```python
from build123d import *

# Parameters (mm, degrees)
SKETCH1_R                    = 16.891
SKETCH1_R_2                  = 7.9375
BOSS_EXTRUDE1_DEPTH          = 12.7
SKETCH2_R                    = 20.6375
CUT_EXTRUDE1_DEPTH           = 7.3914
CHAMFER1_SIZE                = 0.254
SKETCH4_R                    = 2.1844
CUT_EXTRUDE2_DEPTH           = 6.3086
CHAMFER2_SIZE                = 0.254
CIRPATTERN1_COUNT            = 6
CHAMFER2_OF_CIRPATTERN1_SIZE = 0.254


with BuildPart() as part:
    # Sketch1 → Boss-Extrude1 (new body)
    with BuildSketch(Plane(origin=(0, 0, 0), x_dir=(1, 0, 0), z_dir=(0, 1, 0))):
        Circle(SKETCH1_R)
        Circle(SKETCH1_R_2, mode=Mode.SUBTRACT)
    extrude(amount=BOSS_EXTRUDE1_DEPTH)

    # Sketch2 → Cut-Extrude1 (cut)
    with BuildSketch(Plane(origin=(0, 12.7, 0), x_dir=(1, 0, 0), z_dir=(0, 1, 0))):
        Circle(SKETCH2_R)
    extrude(amount=-CUT_EXTRUDE1_DEPTH, mode=Mode.SUBTRACT)

    # Chamfer1
    chamfer1_edges = [part.edges().sort_by_distance(p)[0] for p in [
        (-16.891, 5.3086, 0),
        (-16.891, 0, 0),
    ]]
    chamfer(chamfer1_edges, length=CHAMFER1_SIZE)

    # Sketch3 → Cut-Revolve1 (revolve, cut)
    with BuildSketch(Plane.XY):
        Polygon((-10.7188, 0), (-10.7188, 1.2446), (-9.144, 0.6604), (-9.144, 1.27), (0, 1.27), (0, 0), align=None)
    revolve(axis=Axis((0, 12.7, 0), (0, -1, 0)), mode=Mode.SUBTRACT)

    # Sketch4 → Cut-Extrude2 (cut, through all)
    with BuildSketch(Plane(origin=(0, 5.3086, 0), x_dir=(1, 0, 0), z_dir=(0, 1, 0))):
        with Locations((0, 13.4874)):
            Circle(SKETCH4_R)
    cut_extrude2 = extrude(amount=-CUT_EXTRUDE2_DEPTH, mode=Mode.SUBTRACT)

    # Chamfer2
    chamfer2_edges = [part.edges().sort_by_distance(p)[0] for p in [
        (-2.1844, 0, -13.4874),
        (-2.1844, 5.3086, -13.4874),
    ]]
    chamfer(chamfer2_edges, length=CHAMFER2_SIZE)

    # CirPattern1: Cut-Extrude2 ×6 about axis
    cirpattern1_axis = Axis((0, 0, 0), (0, 1, 0))
    for i in range(1, CIRPATTERN1_COUNT):
        add(cut_extrude2.rotate(cirpattern1_axis, i * 360 / CIRPATTERN1_COUNT), mode=Mode.SUBTRACT)

    # Chamfer2 of CirPattern1
    chamfer2_of_cirpattern1_edges = [part.edges().sort_by_distance(p)[0] for p in [
        (-12.772631031, 0, -4.851954108),
        (-12.772631031, 5.3086, -4.851954108),
        (-10.588231031, 0, 8.635445892),
        (-10.588231031, 5.3086, 8.635445892),
        (2.1844, 0, 13.4874),
        (2.1844, 5.3086, 13.4874),
        (12.772631031, 0, 4.851954108),
        (12.772631031, 5.3086, 4.851954108),
        (10.588231031, 0, -8.635445892),
        (10.588231031, 5.3086, -8.635445892),
    ]]
    chamfer(chamfer2_of_cirpattern1_edges, length=CHAMFER2_OF_CIRPATTERN1_SIZE)


solid = part.part
```
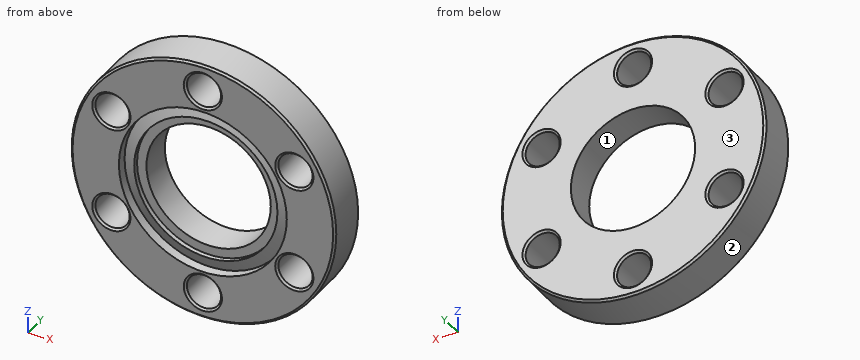
Read the model definition and answer for the solid it produces. Units are mm, in the model's axes. Face numbers are marked on the shaded views. Give positions to 0.01 mm unless a question says otherwise; leave off trailing zeros. Write each loop counter-clockwise with the first axis right and the second up, starting at its lowest first coordinate (ties: lowest second). Pieces come first, ordered by that corner, then holes. Notation, with made-up numbers: M 78.25,-36 L 127.25,-36 A20 ccw 127.25,-1 Z; hole C -14,26.25 d11. An arc over 180 degrees is marked long. Put each result on its own line as item: value. Start each with the question number.
1. The part is cut by section C-C, the plane x = 0. Give the number of separate pieces and of enclosed holes in the cut face, and give its area (3 significant figures).
2. The part is cut by section A-A, the plane z = 0. Give the vertices of the cut face in (x, y), and give its area (3 significant figures).
3. For a pull along Z with two mould halves and no side action, classify the marked faces 1, 2 and 3 as released by +Z, released by -Z, zero draft, split by the parting line, or undercut.
4. The part is cut by section B-B, the plane y = 4.1. Give the vertices of the cut face in (x, z) (1 decimal), and give its area (3 significant figures).
5. Each of these flat-tipped pins is pushed along its axis until it touches: pin 1 Ø3 at (x, z) = (6, -2) entering from +Y; pin 2 Ø1.5 at (x, y) = (-5, 2) entering from +Z; pin 3 Ø2 at (x, y) = (-13.5, 4) entering from -Z; pin 4 Ø6 at (x, z) = (6, -0.5) entering from -Y. Where does it stop, or does it pass through?
6. Consider line 1 along Z through (x, y) = (0, 3.25); line 2 along Z through (x, y) = (-1.5, 3.25); line 3 along Z through (x, y) = (-13, 2.9). Determine where each line is inside the solid, lowest interval first.
Final values:
1. separate pieces: 4
1. enclosed holes: 0
1. area: 42.2 mm²
2. outline: M -16.89,0.25 L -16.64,0 L -10.72,0 L -10.72,1.24 L -9.14,0.66 L -9.14,1.27 L -7.94,1.27 L -7.94,5.31 L -16.64,5.31 L -16.89,5.05 Z; M 7.94,1.27 L 9.14,1.27 L 9.14,0.66 L 10.72,1.24 L 10.72,0 L 16.64,0 L 16.89,0.25 L 16.89,5.05 L 16.64,5.31 L 7.94,5.31 Z
2. area: 88.9 mm²
3. face 1: undercut
3. face 2: split by the parting line
3. face 3: zero draft
4. outline: C 0,0 d33.8; hole C -11.7,-6.7 d4.4; hole C -11.7,6.7 d4.4; hole C 0,0 d15.9; hole C 0,-13.5 d4.4; hole C 0,13.5 d4.4; hole C 11.7,-6.7 d4.4; hole C 11.7,6.7 d4.4
4. area: 608 mm²
5. pin 1: passes through
5. pin 2: stops at z = 16.35
5. pin 3: stops at z = -11.36
5. pin 4: stops at y = 1.27
6. line 1: z = -16.89 to -15.67, -11.3 to -7.94, 7.94 to 11.3, 15.67 to 16.89
6. line 2: z = -16.82 to -15.08, -11.9 to -7.79, 7.79 to 11.9, 15.08 to 16.82
6. line 3: z = -10.78 to -8.48, -5 to 5, 8.48 to 10.78
